Design review of the part built by this model. Coordinates are the model's own, in mm. Face numbers are marked on the shaded views. Give positions to 0.01 mm unless a question says otherwise; leave off trailing zeros. Write each loop counter-clockwise with the first axis right and the second up, starting at its lowest first coordinate (ties: lowest second). Pieces come first, ordered by that corner, then holes. Notation, with made-up numbers: (19.5, 33.5) -> (27.5, 33.5) arc R23 cw to (27.5, 42.5) -> close; hole circle Ø7 at (80, 14). An arc over 180 degrees is marked (long way). Use CSV: the item, a comma, the result in double quotes.
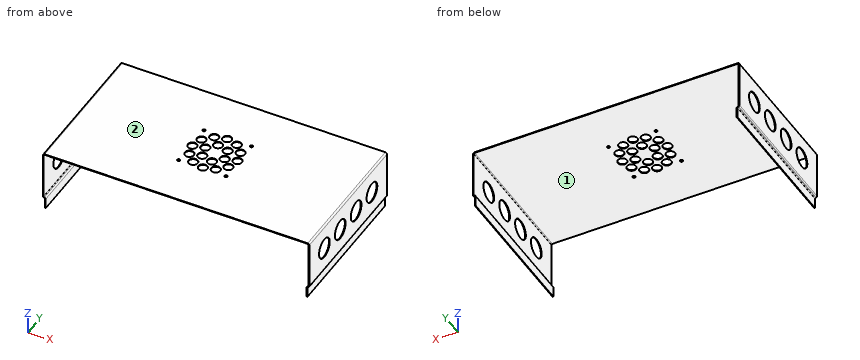
```python
from build123d import *

# Parameters (mm, degrees)
BASE_FLANGE1_DEPTH = 152.4
JOG1_DEPTH         = 152.4
JOG1_2_DEPTH       = 152.4
JOG2_DEPTH         = 152.4
JOG2_2_DEPTH       = 152.4
SKETCH6_R          = 10.5
CUT_EXTRUDE1_DEPTH = 326.842676171
CUT_EXTRUDE4_REACH = 327.337
SKETCH8_R          = 4.7625
CIRPATTERN1_COUNT  = 12
CUT_EXTRUDE5_REACH = 327.337
SKETCH9_R          = 4.7625
CIRPATTERN2_COUNT  = 6
CUT_EXTRUDE6_REACH = 327.337
SKETCH10_R         = 1.5


# Read off the part's stored shape, not the designer's step: Jog1, Jog2
# Sheet-metal steps are written as plain solids
with BuildPart() as part:
    # Sketch1 → Base-Flange1 (new body)
    with BuildSketch(Plane(origin=(0, 0, 0), x_dir=(1, 0, 0), z_dir=(0, 1, 0))):
        with BuildLine():
            Line((0, 63.5), (0, 1))
            ThreePointArc((0, 1), (0.292893219, 0.292893219), (1, 0))
            Line((1, 0), (278.4, 0))
            ThreePointArc((278.4, 0), (279.107106781, 0.292893219), (279.4, 1))
            Line((279.4, 1), (279.4, 63.5))
            Line((279.4, 63.5), (280.15946, 63.5))
            Line((280.15946, 63.5), (280.15946, 1))
            ThreePointArc((280.15946, 1), (279.644126097, -0.244126097), (278.4, -0.75946))
            Line((278.4, -0.75946), (1, -0.75946))
            ThreePointArc((1, -0.75946), (-0.244126097, -0.244126097), (-0.75946, 1))
            Line((-0.75946, 1), (-0.75946, 63.5))
            Line((-0.75946, 63.5), (0, 63.5))
        make_face()
    extrude(amount=BASE_FLANGE1_DEPTH)

    # Jog1 outline → Jog1 (cut)
    with BuildSketch(Plane(origin=(0, 0, 0), x_dir=(1, 0, 0), z_dir=(0, 1, 0))):
        with BuildLine():
            Line((279.4, 63.5), (279.4, 51.344621925))
            ThreePointArc((279.4, 51.344621925), (279.958069237, 50.714354749), (280.15946, 49.896968827))
            Line((280.15946, 49.896968827), (280.15946, 63.5))
            Line((280.15946, 63.5), (279.4, 63.5))
        make_face()
    extrude(amount=JOG1_DEPTH, mode=Mode.SUBTRACT)

    # Jog1 2 outline → Jog1 2 (add)
    with BuildSketch(Plane(origin=(0, 0, 0), x_dir=(1, 0, 0), z_dir=(0, 1, 0))):
        with BuildLine():
            Line((278.114200802, 52.562402507), (278.114200802, 63.5))
            Line((278.114200802, 63.5), (277.354740802, 63.5))
            Line((277.354740802, 63.5), (277.354740802, 52.562402507))
            ThreePointArc((277.354740802, 52.562402507), (277.718327334, 51.491311123), (278.658819045, 50.862894653))
            ThreePointArc((278.658819045, 50.862894653), (279.19335334, 50.505730256), (279.4, 49.896968827))
            Line((279.4, 49.896968827), (279.4, 51.344621925))
            ThreePointArc((279.4, 51.344621925), (279.138506411, 51.493937133), (278.855381757, 51.596476681))
            ThreePointArc((278.855381757, 51.596476681), (278.320847462, 51.953641078), (278.114200802, 52.562402507))
        make_face()
    extrude(amount=JOG1_2_DEPTH)

    # Jog2 outline → Jog2 (cut)
    with BuildSketch(Plane(origin=(0, 0, 0), x_dir=(1, 0, 0), z_dir=(0, 1, 0))):
        with BuildLine():
            ThreePointArc((-0.75946, 49.896968827), (-0.558069237, 50.714354749), (0, 51.344621925))
            Line((0, 51.344621925), (0, 63.5))
            Line((0, 63.5), (-0.75946, 63.5))
            Line((-0.75946, 63.5), (-0.75946, 49.896968827))
        make_face()
    extrude(amount=JOG2_DEPTH, mode=Mode.SUBTRACT)

    # Jog2 2 outline → Jog2 2 (add)
    with BuildSketch(Plane(origin=(0, 0, 0), x_dir=(1, 0, 0), z_dir=(0, 1, 0))):
        with BuildLine():
            Line((2.045259198, 52.562402507), (2.045259198, 63.5))
            Line((2.045259198, 63.5), (1.285799198, 63.5))
            Line((1.285799198, 63.5), (1.285799198, 52.562402507))
            ThreePointArc((1.285799198, 52.562402507), (1.079152538, 51.953641078), (0.544618243, 51.596476681))
            ThreePointArc((0.544618243, 51.596476681), (0.261493589, 51.493937133), (0, 51.344621925))
            Line((0, 51.344621925), (0, 49.896968827))
            ThreePointArc((0, 49.896968827), (0.20664666, 50.505730256), (0.741180955, 50.862894653))
            ThreePointArc((0.741180955, 50.862894653), (1.681672666, 51.491311123), (2.045259198, 52.562402507))
        make_face()
    extrude(amount=JOG2_2_DEPTH)

    # Sketch6 → Cut-Extrude1 (cut, through all)
    with BuildSketch(Plane(origin=(280.15946, 0, 0), x_dir=(0, 0, -1), z_dir=(1, 0, 0))):
        with Locations((25.448484413, 122.85)):
            Circle(SKETCH6_R)
        with Locations((25.448484413, 91.75)):
            Circle(SKETCH6_R)
        with Locations((25.448484413, 60.65)):
            Circle(SKETCH6_R)
        with Locations((25.448484413, 29.55)):
            Circle(SKETCH6_R)
    extrude(amount=-CUT_EXTRUDE1_DEPTH, mode=Mode.SUBTRACT)

    # Sketch8 → Cut-Extrude4 (cut, up to next)
    with BuildSketch(Plane.XY.offset(0.75946), mode=Mode.PRIVATE) as cut_extrude4_sk1:
        with Locations((139.7, 100.0125)):
            Circle(SKETCH8_R)
    cut_extrude4_tool1 = extrude(cut_extrude4_sk1.sketch, amount=-CUT_EXTRUDE4_REACH, mode=Mode.PRIVATE) & part.part
    cut_extrude4 = cut_extrude4_tool1.solids().sort_by_distance((139.7, 100.0125, 0.75946))[0]
    add(cut_extrude4, mode=Mode.SUBTRACT)

    # CirPattern1: Cut-Extrude4 ×12 about axis
    cirpattern1_axis = Axis((139.7, 76.2, 0), (0, 0, 1))
    for i in range(1, CIRPATTERN1_COUNT):
        add(cut_extrude4.rotate(cirpattern1_axis, i * 360 / CIRPATTERN1_COUNT), mode=Mode.SUBTRACT)

    # Sketch9 → Cut-Extrude5 (cut, up to next)
    with BuildSketch(Plane.XY.offset(0.75946), mode=Mode.PRIVATE) as cut_extrude5_sk1:
        with Locations((136.509729928, 88.10625)):
            Circle(SKETCH9_R)
    cut_extrude5_tool1 = extrude(cut_extrude5_sk1.sketch, amount=-CUT_EXTRUDE5_REACH, mode=Mode.PRIVATE) & part.part
    cut_extrude5 = cut_extrude5_tool1.solids().sort_by_distance((136.50973, 88.10625, 0.75946))[0]
    add(cut_extrude5, mode=Mode.SUBTRACT)

    # CirPattern2: Cut-Extrude5 ×6 about axis
    cirpattern2_axis = Axis((139.7, 76.2, 0), (0, 0, 1))
    for i in range(1, CIRPATTERN2_COUNT):
        add(cut_extrude5.rotate(cirpattern2_axis, i * 360 / CIRPATTERN2_COUNT), mode=Mode.SUBTRACT)

    # Sketch10 → Cut-Extrude6 (cut, up to next)
    with BuildSketch(Plane.XY.offset(0.75946), mode=Mode.PRIVATE) as cut_extrude6_sk1:
        with Locations((114.7, 51.2)):
            Circle(SKETCH10_R)
    cut_extrude6_tool1 = extrude(cut_extrude6_sk1.sketch, amount=-CUT_EXTRUDE6_REACH, mode=Mode.PRIVATE) & part.part
    # Sketch10 → Cut-Extrude6 (cut, up to next)
    with BuildSketch(Plane.XY.offset(0.75946), mode=Mode.PRIVATE) as cut_extrude6_sk2:
        with Locations((114.7, 101.2)):
            Circle(SKETCH10_R)
    cut_extrude6_tool2 = extrude(cut_extrude6_sk2.sketch, amount=-CUT_EXTRUDE6_REACH, mode=Mode.PRIVATE) & part.part
    # Sketch10 → Cut-Extrude6 (cut, up to next)
    with BuildSketch(Plane.XY.offset(0.75946), mode=Mode.PRIVATE) as cut_extrude6_sk3:
        with Locations((164.7, 101.2)):
            Circle(SKETCH10_R)
    cut_extrude6_tool3 = extrude(cut_extrude6_sk3.sketch, amount=-CUT_EXTRUDE6_REACH, mode=Mode.PRIVATE) & part.part
    # Sketch10 → Cut-Extrude6 (cut, up to next)
    with BuildSketch(Plane.XY.offset(0.75946), mode=Mode.PRIVATE) as cut_extrude6_sk4:
        with Locations((164.7, 51.2)):
            Circle(SKETCH10_R)
    cut_extrude6_tool4 = extrude(cut_extrude6_sk4.sketch, amount=-CUT_EXTRUDE6_REACH, mode=Mode.PRIVATE) & part.part
    add(cut_extrude6_tool1.solids().sort_by_distance((114.7, 51.2, 0.75946))[0], mode=Mode.SUBTRACT)
    add(cut_extrude6_tool2.solids().sort_by_distance((114.7, 101.2, 0.75946))[0], mode=Mode.SUBTRACT)
    add(cut_extrude6_tool3.solids().sort_by_distance((164.7, 101.2, 0.75946))[0], mode=Mode.SUBTRACT)
    add(cut_extrude6_tool4.solids().sort_by_distance((164.7, 51.2, 0.75946))[0], mode=Mode.SUBTRACT)


solid = part.part
```
(1) Mouldability with a two-part tool opening along X and no side actions: class the marked faces 1 and 2 as +X half, -X half, draft (parallel to the pull), parting line (faces both ways), or undercut.
Established:
face 1,"undercut"
face 2,"draft"
(2) Take a section at A-A (y = 29.55). State how many separate pieces and enclosed holes the cut face has, then the cut area to 3 significant figures.
Established:
separate pieces,"3"
enclosed holes,"0"
area,"278 mm2"
(3) Clearance check with flat-ended pins moving along their axes: pin 1 (12 mm diameter, centred on x = 97.5, y = 64.5, fed in from -Z); pin 2 (7.5 mm diameter, centred on x = 119.08, y = 88.11, fed in from +Z); pin 3 (12.5 mm diameter, centred on x = 151.61, y = 73.01, fed in from +Z); pin 4 (12 mm diameter, centred on y = 83, z = -58, fed in from -X). State where each tip first meets the part, or that it passes through.
Established:
pin 1,"stops at z = 0"
pin 2,"passes through"
pin 3,"stops at z = 0.76"
pin 4,"stops at x = 1.11"
(4) Take a section at B-B (y = 10). Write out the cut boundary in (x, z).
Established:
outline,"(-0.76, -49.9) arc R1.76 ccw to (0.54, -51.6) arc R1 cw to (1.29, -52.56) -> (1.29, -63.5) -> (2.05, -63.5) -> (2.05, -52.56) arc R1.76 ccw to (0.74, -50.86) arc R1 cw to (0, -49.9) -> (0, -1) arc R1 cw to (1, 0) -> (278.4, 0) arc R1 cw to (279.4, -1) -> (279.4, -49.9) arc R1 cw to (278.66, -50.86) arc R1.76 ccw to (277.35, -52.56) -> (277.35, -63.5) -> (278.11, -63.5) -> (278.11, -52.56) arc R1 cw to (278.86, -51.6) arc R1.76 ccw to (280.16, -49.9) -> (280.16, -1) arc R1.76 ccw to (278.4, 0.76) -> (1, 0.76) arc R1.76 ccw to (-0.76, -1) -> close"
(5) For line 1 along X through (y, z) = (83, -46); line 2 along X through (y, z) = (29.5, -58); line 3 along Y through (x, z) = (114.7, 0.65), list the stretches that pass through material, from the lowest coordinate up. Write a range as [from, to].
Established:
line 1,"x = [-0.76, 0], [279.4, 280.16]"
line 2,"x = [1.29, 2.05], [277.35, 278.11]"
line 3,"y = [0, 49.7], [52.7, 62.42], [66.17, 71.59], [80.81, 86.23], [89.98, 99.7], [102.7, 152.4]"
(6) Take a section at D-D (x = 193). Write out the cut boundary in (y, z).
Established:
outline,"(0, 0) -> (152.4, 0) -> (152.4, 0.76) -> (0, 0.76) -> close"
